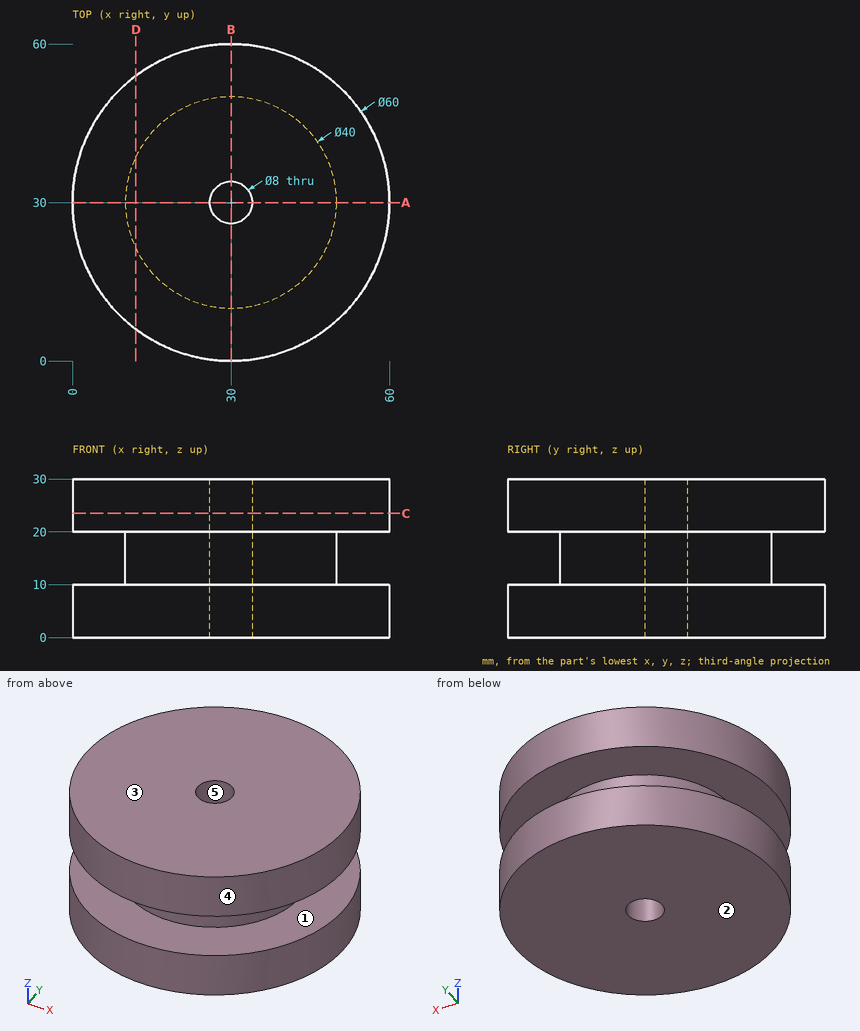
Answer from the drawing. Dimensions are ordinates in mm from the lowest x, y and z of the part. A direction names the side the tool comes from. Give positions to 0.01 mm unless a question says otherwise; leave off trailing zeros. Write each loop counter-clockwise with the first axis right and the second up, starting at its lowest first coordinate (ties: lowest second). Pieces come first, ordered by that corner, then holes. Notation, with made-up numbers: (78.25, 8.25) -> (85.25, 8.25) arc R19 cw to (85.25, 25.25) -> close; hole circle Ø1 at (42.5, -38.5). An arc over 180 degrees is marked (long way). One line per question, with ' | ' between items. Start each with the question number.
1. For the marked faces 1 and 2, determine the directions among +Z, -Z, +X, -X, +Y, -Y from which every point of the face is accessible in a straight line to the end or side of a thin tool.
2. Section A-A (y = 30) is taken. Determine the outline of the cut face in (x, z).
3. For a pull along Y with two mould halves and no side action, classify the marked faces 3, 4 and 5 as pulls with the +Y half, pulls with the -Y half, needs draft (parallel to the pull), parting line crosses it, or undercut.
4. Section D-D (x = 12) is taken. Determine the outline of the cut face in (y, z).
5. Given pin 1 Ø4 at (x, z) = (48, 23.5) entering from +Y; pin 2 Ø5 at (y, z) = (17, 20.5) entering from -X; pin 3 Ø1 at (x, z) = (33.5, 22) entering from -Y, each flat-ended and moving along its own axis, determine where each tip first touches the part or whether it passes through.
6. Find the intervals of material crossed by probe 1 along Z at (x, y) = (4, 27); probe 2 along Y at (x, z) = (30, 19.75); probe 3 along Y at (x, z) = (27, 23.25), in increasing order.
7. Section C-C (z = 23.5) is taken. Determine the outline of the cut face in (x, y), plus the area to 3 significant figures.
Response values:
1) face 1: none | face 2: -Z, +X, -X, +Y, -Y
2) outline: (0, 0) -> (26, 0) -> (26, 30) -> (0, 30) -> (0, 20) -> (10, 20) -> (10, 10) -> (0, 10) -> close; (34, 0) -> (60, 0) -> (60, 10) -> (50, 10) -> (50, 20) -> (60, 20) -> (60, 30) -> (34, 30) -> close
3) face 3: needs draft | face 4: parting line crosses it | face 5: undercut
4) outline: (6, 0) -> (54, 0) -> (54, 10) -> (38.72, 10) -> (38.72, 20) -> (54, 20) -> (54, 30) -> (6, 30) -> (6, 20) -> (21.28, 20) -> (21.28, 10) -> (6, 10) -> close
5) pin 1: y = 55.38 | pin 2: x = 1.9 | pin 3: y = 0.15
6) probe 1: 0 to 10, 20 to 30 | probe 2: 10 to 26, 34 to 50 | probe 3: 0.15 to 27.35, 32.65 to 59.85
7) outline: circle Ø60 at (30, 30); hole circle Ø8 at (30, 30) | area: 2,780 mm2
